Verification items for the finished model (mm, model axes). A direction names the side the tool comes from. Coordinates: 2 decimals unless noted, no trailing zeros. Write each loop counter-clockwise with the first axis right and the second up, starting at its lowest first coordinate (ties: lowest second). Pieces come first, ordered by that corner, then holes. Notation, with made-up numbers: (15, 18) -> (47, 18) arc R34 ccw to (47, 51) -> close; hole circle Ø9 at (48.5, -13.5). An arc over 180 degrees is marked (long way). Use CSV: the item, a comma, the result in double quotes.
```python
from build123d import *

# Parameters (mm, degrees)
SALIENTE_EXTRUIR1_DEPTH = 40
CORTAR_EXTRUIR1_REACH   = 25.383
CROQUIS2_R              = 6.25
REDONDEO1_R             = 10
CORTAR_EXTRUIR2_REACH   = 110.313
CROQUIS3_R              = 2.3
CORTAR_EXTRUIR3_REACH   = 95.802
CROQUIS4_R              = 1.75
CORTAR_EXTRUIR4_REACH   = 89.802
CROQUIS5_R              = 3.5


with BuildPart() as part:
    # Croquis1 → Saliente-Extruir1 (new body)
    with BuildSketch(Plane.XY):
        Polygon((80.813466521, 8.767949192), (-13.999287239, 8.767949192), (-13.999287239, 32.150635095), (94.313466521, 32.150635095), align=None)
    extrude(amount=SALIENTE_EXTRUIR1_DEPTH)

    # Croquis2 → Cortar-Extruir1 (cut, up to next)
    with BuildSketch(Plane(origin=(0, 32.150635095, 0), x_dir=(1, 0, 0), z_dir=(0, 1, 0)), mode=Mode.PRIVATE) as cortar_extruir1_sk1:
        with Locations((0, -20)):
            Circle(CROQUIS2_R)
    cortar_extruir1_tool1 = extrude(cortar_extruir1_sk1.sketch, amount=-CORTAR_EXTRUIR1_REACH, mode=Mode.PRIVATE) & part.part
    add(cortar_extruir1_tool1.solids().sort_by_distance((0, 32.150635, 20))[0], mode=Mode.SUBTRACT)

    # Redondeo1
    redondeo1_edges = [part.edges().sort_by_distance(p)[0] for p in [
        (-13.999287239, 20.459292144, 0),
        (-13.999287239, 20.459292144, 40),
    ]]
    fillet(redondeo1_edges, radius=REDONDEO1_R)

    # Croquis3 → Cortar-Extruir2 (cut, up to next)
    with BuildSketch(Plane.ZY.offset(13.999287239), mode=Mode.PRIVATE) as cortar_extruir2_sk1:
        with Locations((20, 20.150635095)):
            Circle(CROQUIS3_R)
    cortar_extruir2_tool1 = extrude(cortar_extruir2_sk1.sketch, amount=-CORTAR_EXTRUIR2_REACH, mode=Mode.PRIVATE) & part.part
    add(cortar_extruir2_tool1.solids().sort_by_distance((-13.999287, 20.150635, 20))[0], mode=Mode.SUBTRACT)

    # Croquis4 → Cortar-Extruir3 (cut, up to next)
    with BuildSketch(Plane(origin=(56.813466521, -32.801270189, 0), x_dir=(0, 0, -1), z_dir=(0.866025404, -0.5, 0)), mode=Mode.PRIVATE) as cortar_extruir3_sk1:
        with Locations((-30, 54)):
            Circle(CROQUIS4_R)
    cortar_extruir3_tool1 = extrude(cortar_extruir3_sk1.sketch, amount=-CORTAR_EXTRUIR3_REACH, mode=Mode.PRIVATE) & part.part
    add(cortar_extruir3_tool1.solids().sort_by_distance((83.813467, 13.964102, 30))[0], mode=Mode.SUBTRACT)
    # Croquis4 → Cortar-Extruir3 (cut, up to next)
    with BuildSketch(Plane(origin=(56.813466521, -32.801270189, 0), x_dir=(0, 0, -1), z_dir=(0.866025404, -0.5, 0)), mode=Mode.PRIVATE) as cortar_extruir3_sk2:
        with Locations((-10, 54)):
            Circle(CROQUIS4_R)
    cortar_extruir3_tool2 = extrude(cortar_extruir3_sk2.sketch, amount=-CORTAR_EXTRUIR3_REACH, mode=Mode.PRIVATE) & part.part
    add(cortar_extruir3_tool2.solids().sort_by_distance((83.813467, 13.964102, 10))[0], mode=Mode.SUBTRACT)
    # Croquis4 → Cortar-Extruir3 (cut, up to next)
    with BuildSketch(Plane(origin=(56.813466521, -32.801270189, 0), x_dir=(0, 0, -1), z_dir=(0.866025404, -0.5, 0)), mode=Mode.PRIVATE) as cortar_extruir3_sk3:
        with Locations((-20, 67)):
            Circle(CROQUIS4_R)
    cortar_extruir3_tool3 = extrude(cortar_extruir3_sk3.sketch, amount=-CORTAR_EXTRUIR3_REACH, mode=Mode.PRIVATE) & part.part
    add(cortar_extruir3_tool3.solids().sort_by_distance((90.313467, 25.222432, 20))[0], mode=Mode.SUBTRACT)

    # Croquis5 → Cortar-Extruir4 (cut, up to next)
    with BuildSketch(Plane(origin=(51.617314098, -29.801270189, 0), x_dir=(0, 0, -1), z_dir=(0.866025404, -0.5, 0)), mode=Mode.PRIVATE) as cortar_extruir4_sk1:
        with Locations((-30, 54)):
            Circle(CROQUIS5_R)
    cortar_extruir4_tool1 = extrude(cortar_extruir4_sk1.sketch, amount=-CORTAR_EXTRUIR4_REACH, mode=Mode.PRIVATE) & part.part
    add(cortar_extruir4_tool1.solids().sort_by_distance((78.617314, 16.964102, 30))[0], mode=Mode.SUBTRACT)
    # Croquis5 → Cortar-Extruir4 (cut, up to next)
    with BuildSketch(Plane(origin=(51.617314098, -29.801270189, 0), x_dir=(0, 0, -1), z_dir=(0.866025404, -0.5, 0)), mode=Mode.PRIVATE) as cortar_extruir4_sk2:
        with Locations((-20, 67)):
            Circle(CROQUIS5_R)
    cortar_extruir4_tool2 = extrude(cortar_extruir4_sk2.sketch, amount=-CORTAR_EXTRUIR4_REACH, mode=Mode.PRIVATE) & part.part
    add(cortar_extruir4_tool2.solids().sort_by_distance((85.117314, 28.222432, 20))[0], mode=Mode.SUBTRACT)
    # Croquis5 → Cortar-Extruir4 (cut, up to next)
    with BuildSketch(Plane(origin=(51.617314098, -29.801270189, 0), x_dir=(0, 0, -1), z_dir=(0.866025404, -0.5, 0)), mode=Mode.PRIVATE) as cortar_extruir4_sk3:
        with Locations((-10, 54)):
            Circle(CROQUIS5_R)
    cortar_extruir4_tool3 = extrude(cortar_extruir4_sk3.sketch, amount=-CORTAR_EXTRUIR4_REACH, mode=Mode.PRIVATE) & part.part
    add(cortar_extruir4_tool3.solids().sort_by_distance((78.617314, 16.964102, 10))[0], mode=Mode.SUBTRACT)


solid = part.part
```
1) Cross-section at A-A (x = 0). Record the boundary of the cut face in (y, z), plus the area to 3 significant figures.
Return value:
outline,"(8.77, 0) -> (32.15, 0) -> (32.15, 13.75) -> (8.77, 13.75) -> close; (8.77, 26.25) -> (32.15, 26.25) -> (32.15, 40) -> (8.77, 40) -> close"
area,"643 mm2"
2) Gauge pin test, flat ends, axial feed: pin 1 (7.5 mm diameter, centred on x = 0, z = 20, fed in from +Y); pin 2 (12 mm diameter, centred on y = 26, z = 6.5, fed in from +X); pin 3 (5 mm diameter, centred on y = 28.5, z = 7.5, fed in from +X); pin 4 (8 mm diameter, centred on y = 12.5, z = 28.5, fed in from +X). Record the tip position at first contact, or that the pin passes through.
Return value:
pin 1,"through"
pin 2,"x = 94.23"
pin 3,"x = 93.65"
pin 4,"x = 85.28"
3) Cross-section at C-C (x = 75.5). Give the number of separate pieces and of enclosed holes in the cut face, plus the area to 3 significant figures.
Return value:
separate pieces,"1"
enclosed holes,"2"
area,"835 mm2"
4) Scan lines: L1, parallel to Y at x = -10, z = 20; L2, parallel to Z at x = 69.5, y = 23.5; L3, parallel to Z at x = 74, y = 22.75. Record each from-to range of solid material in increasing order.
Return value:
L1,"8.77 to 17.85, 22.45 to 32.15"
L2,"0 to 6.68, 13.32 to 26.68, 33.32 to 40"
L3,"0 to 7.78, 12.22 to 27.78, 32.22 to 40"
5) Set-up check for faces 1 (the flat face through (77.864, 15.659, 28.493)), 2 (the flat face through (46, 21, 40)), 3 (the cylindrical face through (-9.963, 19.27, 22.125)): record each of +Z, -Z, +X, -X, +Y, -Y from which the full face is reachable in a straight line by a thin tool's end or side.
Return value:
face 1,"none"
face 2,"+Z, +X, -X, +Y, -Y"
face 3,"-X"
6) Mould release check, pull along Y, two halves, no side actions. Record for faces 4 (the cylindrical face through (-10.99, 20.62, 2.85)), 5 (the flat face through (39, 32.151, 20)), 6 (the cylindrical face through (80.72, 14.52, 31.39)): released by +Y, released by -Y, zero draft, split by the parting line, or undercut.
Return value:
face 4,"zero draft"
face 5,"released by +Y"
face 6,"undercut"
7) Cross-section at D-D (z = 3). Record the boundary of the cut face in (x, y).
Return value:
outline,"(-11.14, 8.77) -> (80.81, 8.77) -> (94.31, 32.15) -> (-11.14, 32.15) -> close"
8) Cross-section at B-B (z = 20). Record the boundary of the cut face in (x, y), plus the area to 3 significant figures.
Return value:
outline,"(-14, 8.77) -> (-6.25, 8.77) -> (-6.25, 17.85) -> (-14, 17.85) -> close; (-14, 22.45) -> (-6.25, 22.45) -> (-6.25, 32.15) -> (-14, 32.15) -> close; (6.25, 8.77) -> (80.81, 8.77) -> (89.44, 23.71) -> (84.24, 26.71) -> (83.37, 25.19) -> (71.31, 32.15) -> (6.25, 32.15) -> close; (85.31, 32.15) -> (86.87, 31.25) -> (85.99, 29.74) -> (91.19, 26.74) -> (94.31, 32.15) -> close"
area,"1,970 mm2"
